Can you work these out from the model? Positions are in its coordinate system, mm. A direction names the side the tool comes from. Coordinates: 2 decimals unless noted, no trailing zeros. Loops run counter-clockwise (first coordinate to the right, second up) from the corner with the lowest first, then second, coordinate; pieces in that order, holes last.
```python
from build123d import *

# Parameters (mm, degrees)
SKETCH1_R           = 1.5
BOSS_EXTRUDE1_DEPTH = 3
CUT_EXTRUDE1_DEPTH  = 40.962482405


with BuildPart() as part:
    # Sketch1 → Boss-Extrude1 (new body)
    with BuildSketch(Plane.XY):
        with BuildLine():
            Line((0, 0), (32, 0))
            ThreePointArc((32, 0), (38, 6), (32, 12))
            Line((32, 12), (0, 12))
            ThreePointArc((0, 12), (-6, 6), (0, 0))
        make_face()
        with Locations((0, 6)):
            Circle(SKETCH1_R, mode=Mode.SUBTRACT)
        with Locations((32, 6)):
            Circle(SKETCH1_R, mode=Mode.SUBTRACT)
    extrude(amount=BOSS_EXTRUDE1_DEPTH)

    # Sketch2 → Cut-Extrude1 (cut, through all)
    with BuildSketch(Plane.XY.offset(3)):
        with BuildLine():
            Line((3, 9.5), (11, 9.5))
            Line((11, 9.5), (11, 8))
            Line((11, 8), (13.127718677, 8))
            ThreePointArc((13.127718677, 8), (19.5, 6), (13.127718677, 4))
            Line((13.127718677, 4), (11, 4))
            Line((11, 4), (11, 2.5))
            Line((11, 2.5), (3, 2.5))
            Line((3, 2.5), (3, 9.5))
        make_face()
    extrude(amount=-CUT_EXTRUDE1_DEPTH, mode=Mode.SUBTRACT)


solid = part.part
```
(1) If I drill on probe 1 along Y at (x, z) = (0, 2.3); probe 2 along X at (y, z) = (5.5, 2.7); probe 3 along X at (y, z) = (8.5, 1.6), over which ranges is the centre line in solid material (lowest first)?
Check values:
probe 1: y = 0 to 4.5, 7.5 to 12
probe 2: x = -5.98 to -1.41, 1.41 to 3, 19.46 to 30.59, 33.41 to 37.98
probe 3: x = -5.45 to 3, 11 to 13.55, 18.45 to 37.45
(2) I want a section at D-D on y = 6. Write out the boundary of the cut face in (x, z), then the cut area to 3 significant figures.
Check values:
outline: (-6, 0) - (-1.5, 0) - (-1.5, 3) - (-6, 3) - close; (1.5, 0) - (3, 0) - (3, 3) - (1.5, 3) - close; (19.5, 0) - (30.5, 0) - (30.5, 3) - (19.5, 3) - close; (33.5, 0) - (38, 0) - (38, 3) - (33.5, 3) - close
area: 64.5 mm2
(3) Which directions (+Z, -Z, +X, -X, +Y, -Y) give clear straight access to the entire face, cutting with the end or side of a thin tool? Please do faces 1 (the flat face through (7, 2.5, 2)), 2 (the flat face through (21, 6, 0)).
Check values:
face 1: +Z, -Z
face 2: -Z, +X, -X, +Y, -Y
(4) I'm going to push flat-ended pins straight in: pin 1 (0.8 mm diameter, centred on y = 8.5, z = 1, fed in from -X); pin 2 (1.5 mm diameter, centred on x = 14.5, y = 8, fed in from +Z); pin 3 (1.2 mm diameter, centred on y = 3, z = 2, fed in from -X); pin 4 (0.9 mm diameter, centred on y = 5, z = 1, fed in from +X). Where does each tip first touch, or does it pass through?
Check values:
pin 1: stops at x = -5.62
pin 2: passes through
pin 3: stops at x = -5.5
pin 4: stops at x = 37.97
(5) I want a section at A-A on x = 7.5. Write out the boundary of the cut face in (y, z), then the cut area to 3 significant figures.
Check values:
outline: (0, 0) - (2.5, 0) - (2.5, 3) - (0, 3) - close; (9.5, 0) - (12, 0) - (12, 3) - (9.5, 3) - close
area: 15.0 mm2
(6) If we mould it in two halves opening along Y, with no side actions, what happens to faces 3 (the cylindrical face through (30.5, 6.07, 1.48)), 4 (the flat face through (16, 12, 1)), 5 (the cylindrical face through (-6, 6, 1))? For each: released by +Y, released by -Y, zero draft, split by the parting line, or undercut.
Check values:
face 3: undercut
face 4: released by +Y
face 5: split by the parting line
(7) I want a section at C-C on y = 3.25. Write out the boundary of the cut face in (x, z), then the cut area to 3 significant figures.
Check values:
outline: (-5.33, 0) - (3, 0) - (3, 3) - (-5.33, 3) - close; (11, 0) - (13.83, 0) - (13.83, 3) - (11, 3) - close; (18.17, 0) - (37.33, 0) - (37.33, 3) - (18.17, 3) - close
area: 91.0 mm2
(8) I want a section at B-B on z = 1.6. Write out the boundary of the cut face in (x, y), then the cut area to 3 significant figures.
Check values:
outline: (0, 0) - (32, 0) arc R6 ccw to (32, 12) - (0, 12) arc R6 ccw to start; hole circle Ø3 at (0, 6); hole (3, 2.5) - (11, 2.5) - (11, 4) - (13.13, 4) arc R3.5 ccw (long way) to (13.13, 8) - (11, 8) - (11, 9.5) - (3, 9.5) - close; hole circle Ø3 at (32, 6)
area: 382 mm2
